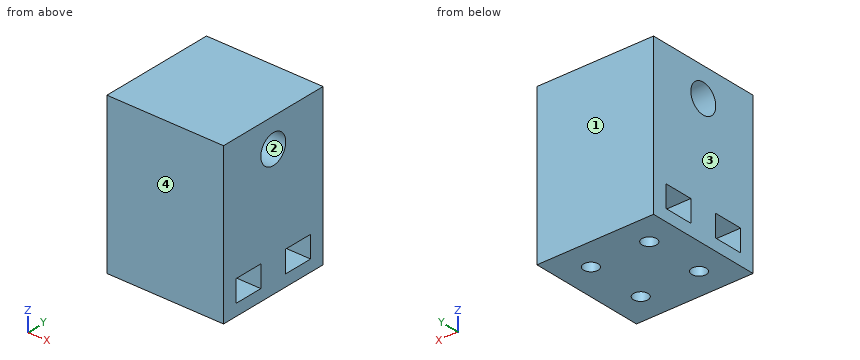
from build123d import *

# Parameters (mm, degrees)
F0_W     = 80
F0_H     = 80
F1_DEPTH = 50
F2_R     = 5
F3_DEPTH = 10
F4_R     = 10
F5_DEPTH = 86.1
F6_W     = 20
F6_H     = 15
F7_DEPTH = 84.6
F2_W     = 80
F2_H     = 80
F8_DEPTH = 8


# Not quite as in the source:
# - a pattern or mirror of a feature is missing from the dataset's text; its kind, count and spacing are read off the source's solid


with BuildPart() as f1:
    # F0 (on Top) → F1 (new body, symmetric)
    with BuildSketch(Plane.XY):
        Rectangle(F0_W, F0_H)
    extrude(amount=F1_DEPTH, both=True)

    # F2 (on face) → F3 (cut)
    with BuildSketch(Plane(origin=(0, 0, -50), x_dir=(1, 0, 0), z_dir=(0, 0, -1))):
        with Locations((-20, 20)):
            Circle(F2_R)
        with Locations((-20, -20)):
            Circle(F2_R)
        with Locations((20, -20)):
            Circle(F2_R)
        with Locations((20, 20)):
            Circle(F2_R)
    extrude(amount=-F3_DEPTH, mode=Mode.SUBTRACT)

    # F4 (on face) → F5 (cut)
    with BuildSketch(Plane(origin=(-40, 0, 0), x_dir=(0, -1, 0), z_dir=(-1, 0, 0))):
        with Locations((0, 30)):
            Circle(F4_R)
    extrude(amount=-F5_DEPTH, mode=Mode.SUBTRACT)

    # F6 (on face) → F7 (cut)
    with BuildSketch(Plane(origin=(-40, 0, 0), x_dir=(0, -1, 0), z_dir=(-1, 0, 0))):
        with Locations((-20, -42.5)):
            Rectangle(F6_W, F6_H)
    f7 = extrude(amount=-F7_DEPTH, mode=Mode.SUBTRACT)

    # F7_copies: F7 across plane
    add(f7.mirror(Plane(origin=(0, 0, 0), x_dir=(0, 0, -1), z_dir=(0, -1, 0))), mode=Mode.SUBTRACT)

    # F2 (on face) → F8 (join)
    with BuildSketch(Plane(origin=(0, 0, -50), x_dir=(1, 0, 0), z_dir=(0, 0, -1))):
        Rectangle(F2_W, F2_H)
        with Locations((-20, -20)):
            Circle(F2_R, mode=Mode.SUBTRACT)
        with Locations((20, -20)):
            Circle(F2_R, mode=Mode.SUBTRACT)
        with Locations((-20, 20)):
            Circle(F2_R, mode=Mode.SUBTRACT)
        with Locations((20, 20)):
            Circle(F2_R, mode=Mode.SUBTRACT)
    extrude(amount=F8_DEPTH)


solid = f1.part
Geometry check sheet. Reference: the model listing, model coordinates, mm. Face numbers are marked on the shaded views. Give positions to 0.01 mm unless a question says otherwise; leave off trailing zeros. Loops run counter-clockwise (first coordinate to the right, second up) from the corner with the lowest first, then second, coordinate; pieces in that order, holes last. Notation, with made-up numbers: M 50,-6 L 57,-6 A24 ccw 57,14 Z; hole C 87.5,84 d11. An arc over 180 degrees is marked long. Answer as a JSON object with one key per item and string values. Group by question number.
Item 1: Material ranges on L1, parallel to X at y = -20, z = -53; L2, parallel to Y at x = 23, z = -48.5, recorded low to high.
Item 2: Gauge pin test, flat end, axial feed: pin 1 (9 mm diameter, centred on x = 20, y = 20, fed in from -Z). Record the tip position at first contact, or that the pin passes through.
Item 3: Sectioned sample at D-D on x = -33.5. Record the boundary of the cut face in (y, z), plus the area to 3 significant figures.
Item 4: Mould release check, pull along Y, two halves, no side actions. Record for the marked faces 1, 2, 3 and 4: pulls with the +Y half, pulls with the -Y half, needs draft (parallel to the pull), parting line crosses it, or undercut.
Item 5: Sectioned sample at A-A on y = 20. Record the boundary of the cut face in (x, z).
Item 6: Sectioned sample at C-C on y = -13. Record the boundary of the cut face in (x, z).
Item 7: Sectioned sample at B-B on x = -20. Record the boundary of the cut face in (y, z).
Findings below:
{
 "1": {"L1": "-40 to -25, -15 to 15, 25 to 40", "L2": "-40 to -30, -10 to 10, 30 to 40"},
 "2": {"pin 1": "z = -35"},
 "3": {"outline": "M -40,-58 L 40,-58 L 40,50 L -40,50 Z; hole M -30,-50 L -10,-50 L -10,-35 L -30,-35 Z; hole C 0,30 d20; hole M 10,-50 L 30,-50 L 30,-35 L 10,-35 Z", "area": "7,730 mm2"},
 "4": {"face 1": "pulls with the +Y half", "face 2": "undercut", "face 3": "needs draft", "face 4": "pulls with the -Y half"},
 "5": {"outline": "M -40,-58 L -25,-58 L -25,-50 L -40,-50 Z; M -40,-35 L 40,-35 L 40,50 L -40,50 Z; M -15,-58 L 15,-58 L 15,-50 L -15,-50 Z; M 25,-58 L 40,-58 L 40,-50 L 25,-50 Z"},
 "6": {"outline": "M -40,-58 L 40,-58 L 40,-50 L -40,-50 Z; M -40,-35 L 40,-35 L 40,50 L -40,50 Z"},
 "7": {"outline": "M -40,-58 L -25,-58 L -25,-50 L -30,-50 L -30,-35 L -10,-35 L -10,-50 L -15,-50 L -15,-58 L 15,-58 L 15,-50 L 10,-50 L 10,-35 L 30,-35 L 30,-50 L 25,-50 L 25,-58 L 40,-58 L 40,50 L -40,50 Z; hole C 0,30 d20"}
}
